Source: CAD feature listing. Evaluate the final solid. Frame: model axes, mm. A direction names the side the tool comes from. Coordinates: 2 decimals unless noted, no trailing zeros. Loops run counter-clockwise (first coordinate to the right, second up) from the corner with the lowest first, then second, coordinate; pieces in that order, holes last.
```python
from build123d import *

# Parameters (mm, degrees)
PAD_DEPTH = 5


with BuildPart() as part:
    # Sketch → Pad (new body, symmetric)
    with BuildSketch(Plane.XY):
        with BuildLine():
            Line((-42.469309, -75), (54.5, -75))
            Line((54.5, -75), (54.5, 75))
            Line((54.5, 75), (-54.5, 75))
            Line((-54.5, 75), (-54.5, -62.969309))
            ThreePointArc((-54.5, -62.969309), (-50.976292, -71.476292), (-42.469309, -75))
        make_face()
        with BuildLine():
            Line((-41.055096, -70), (49.5, -70))
            Line((49.5, -70), (49.5, 70))
            Line((49.5, 70), (-49.5, 70))
            Line((-49.5, 70), (-49.5, -61.555096))
            ThreePointArc((-49.5, -61.555096), (-47.026545, -67.526545), (-41.055096, -70))
        make_face(mode=Mode.SUBTRACT)
    extrude(amount=PAD_DEPTH, both=True)


solid = part.part
```
Q1. Material intervals for line 1 along X through (y, z) = (46, 4.75); line 2 along Y through (x, z) = (-36, -2.75); line 3 along X through (y, z) = (-64, -3), sorted ascending.
Q2. Draft query along Y for faces 3 (the flat face through (1, 75, 0)), 4 (the flat face through (49.5, -1, 0)), 5 (the flat face through (-53, 0, 5)). Return one class per face: released by +Y, released by -Y, zero draft, split by the parting line, or undercut.
Q3. Reachability of faces 1 (the flat face through (4, -70, 0)), 2 (the flat face through (-54.5, 7, 0)) from +Z, -Z, +X, -X, +Y, -Y: full face, straight path, thin tool, end or side. Return the list, or none.
Q4. Section query A-A on y = -32. Return the cut outline in (x, z).
Q5. Section query B-B on x = -39. Return the cut outline in (y, z).
Q6. Section query C-C on z = 2.25. Return the cut outline in (x, y), then the cut area to 3 significant figures.
Resolved:
1. line 1: x = -54.5 to -49.5, 49.5 to 54.5
1. line 2: y = -75 to -70, 70 to 75
1. line 3: x = -54.46 to -49.14, 49.5 to 54.5
2. face 3: released by +Y
2. face 4: undercut
2. face 5: zero draft
3. face 1: +Z, -Z
3. face 2: +Z, -Z, -X, +Y, -Y
4. outline: (-54.5, -5) - (-49.5, -5) - (-49.5, 5) - (-54.5, 5) - close; (49.5, -5) - (54.5, -5) - (54.5, 5) - (49.5, 5) - close
5. outline: (-75, -5) - (-70, -5) - (-70, 5) - (-75, 5) - close; (70, -5) - (75, -5) - (75, 5) - (70, 5) - close
6. outline: (-54.5, -62.97) arc R12.03 ccw to (-42.47, -75) - (54.5, -75) - (54.5, 75) - (-54.5, 75) - close; hole (-49.5, -61.56) arc R8.44 ccw to (-41.06, -70) - (49.5, -70) - (49.5, 70) - (-49.5, 70) - close
6. area: 2,470 mm2
